Source: CAD feature listing. Evaluate the final solid. Frame: model axes, mm. A direction names the side the tool comes from. Give positions to 0.01 mm unless a question says otherwise; leave off trailing zeros. Order: outer loops, then holes, each group sorted by start corner. A loop starts at its lowest first (then second) coordinate and runs counter-clockwise, first axis right, second up.
```python
from build123d import *

# Parameters (mm, degrees)
BASE_FLANGE1_DEPTH      = 60
SKETCH6_R               = 15
CUT_EXTRUDE1_DEPTH      = 3.4
CUT_EXTRUDE2_START      = -65
CUT_EXTRUDE2_OUTLINE_W  = 10
CUT_EXTRUDE2_OUTLINE_H  = 10.4
CUT_EXTRUDE2_DEPTH      = 50
SKETCH10_W              = 3
SKETCH10_H              = 3.4
BOSS_EXTRUDE1_DEPTH     = 30
MIRROR2_COPY_1_SKETCH_W = 3
MIRROR2_COPY_1_SKETCH_H = 3.4
MIRROR2_COPY_1_DEPTH    = 30
SKETCH13_R              = 1.5
CUT_EXTRUDE3_DEPTH      = 141.516902898
CUT_EXTRUDE6_REACH      = 142.517
SKETCH14_R              = 2.5
CUT_EXTRUDE7_START      = -3.4
CUT_EXTRUDE7_DEPTH      = 10.4


# Read off the part's stored shape, not the designer's step: Cut-Extrude2
# Sheet-metal steps are written as plain solids
with BuildPart() as part:
    # Sketch1 → Base-Flange1 (new body)
    with BuildSketch(Plane.XY):
        with BuildLine():
            Line((100, 0), (4.4, 0))
            ThreePointArc((4.4, 0), (1.288730163, -1.288730163), (0, -4.4))
            Line((0, -4.4), (0, -71.6))
            ThreePointArc((0, -71.6), (1.288730163, -74.711269837), (4.4, -76))
            Line((4.4, -76), (45.6, -76))
            ThreePointArc((45.6, -76), (48.711269837, -74.711269837), (50, -71.6))
            Line((50, -71.6), (50, -70))
            ThreePointArc((50, -70), (50.292893219, -69.292893219), (51, -69))
            Line((51, -69), (100, -69))
            Line((100, -69), (100, -65.6))
            Line((100, -65.6), (51, -65.6))
            ThreePointArc((51, -65.6), (47.888730163, -66.888730163), (46.6, -70))
            Line((46.6, -70), (46.6, -71.6))
            ThreePointArc((46.6, -71.6), (46.307106781, -72.307106781), (45.6, -72.6))
            Line((45.6, -72.6), (4.4, -72.6))
            ThreePointArc((4.4, -72.6), (3.692893219, -72.307106781), (3.4, -71.6))
            Line((3.4, -71.6), (3.4, -4.4))
            ThreePointArc((3.4, -4.4), (3.692893219, -3.692893219), (4.4, -3.4))
            Line((4.4, -3.4), (100, -3.4))
            Line((100, -3.4), (100, 0))
        make_face()
    extrude(amount=BASE_FLANGE1_DEPTH)

    # Sketch6 → Cut-Extrude1 (cut)
    with BuildSketch(Plane.ZY):
        with Locations(Location((30, -50, 0), (0, 0, 270))):
            Circle(SKETCH6_R)
        with BuildLine():
            Line((57.224873734, -63.689339828), (55.810660172, -62.275126266))
            ThreePointArc((55.810660172, -62.275126266), (52.275126266, -62.275126266), (52.275126266, -65.810660172))
            Line((52.275126266, -65.810660172), (53.689339828, -67.224873734))
            ThreePointArc((53.689339828, -67.224873734), (57.224873734, -67.224873734), (57.224873734, -63.689339828))
        make_face()
        with BuildLine():
            Line((2.775126266, -16.310660172), (4.189339828, -17.724873734))
            ThreePointArc((4.189339828, -17.724873734), (7.724873734, -17.724873734), (7.724873734, -14.189339828))
            Line((7.724873734, -14.189339828), (6.310660172, -12.775126266))
            ThreePointArc((6.310660172, -12.775126266), (2.775126266, -12.775126266), (2.775126266, -16.310660172))
        make_face()
        with BuildLine():
            Line((53.689339828, -12.775126266), (52.275126266, -14.189339828))
            ThreePointArc((52.275126266, -14.189339828), (52.275126266, -17.724873734), (55.810660172, -17.724873734))
            Line((55.810660172, -17.724873734), (57.224873734, -16.310660172))
            ThreePointArc((57.224873734, -16.310660172), (57.224873734, -12.775126266), (53.689339828, -12.775126266))
        make_face()
        with BuildLine():
            Line((6.310660172, -67.224873734), (7.724873734, -65.810660172))
            ThreePointArc((7.724873734, -65.810660172), (7.724873734, -62.275126266), (4.189339828, -62.275126266))
            Line((4.189339828, -62.275126266), (2.775126266, -63.689339828))
            ThreePointArc((2.775126266, -63.689339828), (2.775126266, -67.224873734), (6.310660172, -67.224873734))
        make_face()
    extrude(amount=-CUT_EXTRUDE1_DEPTH, mode=Mode.SUBTRACT)

    # Cut-Extrude2 outline → Cut-Extrude2 (cut)
    with BuildSketch(Plane.ZY.offset(CUT_EXTRUDE2_START)):
        with Locations((55, -70.8)):
            Rectangle(CUT_EXTRUDE2_OUTLINE_W, CUT_EXTRUDE2_OUTLINE_H)
        with Locations((5, -70.8)):
            Rectangle(CUT_EXTRUDE2_OUTLINE_W, CUT_EXTRUDE2_OUTLINE_H)
    extrude(amount=CUT_EXTRUDE2_DEPTH, mode=Mode.SUBTRACT)

    # Sketch10 → Boss-Extrude1 (add)
    with BuildSketch(Plane(origin=(100, 0, 0), x_dir=(0, 0, -1), z_dir=(1, 0, 0))):
        with Locations((1.5, -1.7)):
            Rectangle(SKETCH10_W, SKETCH10_H)
    boss_extrude1 = extrude(amount=-BOSS_EXTRUDE1_DEPTH)

    # Mirror1: Boss-Extrude1 across plane
    add(boss_extrude1.mirror(Plane(origin=(0, 0, 30), x_dir=(1, 0, 0), z_dir=(0, 0, -1))))

    # Mirror2: Boss-Extrude1 across plane
    add(boss_extrude1.mirror(Plane(origin=(0, -34.5, 0), x_dir=(0, 0, 1), z_dir=(0, -1, 0))))

    # Mirror2 copy 1 sketch → Mirror2 copy 1 (add)
    with BuildSketch(Plane(origin=(100, -69, 60), x_dir=(0, 0, 1), z_dir=(1, 0, 0))):
        with Locations((1.5, -1.7)):
            Rectangle(MIRROR2_COPY_1_SKETCH_W, MIRROR2_COPY_1_SKETCH_H)
    extrude(amount=-MIRROR2_COPY_1_DEPTH)

    # Sketch13 → Cut-Extrude3 (cut, through all)
    with BuildSketch(Plane(origin=(0, 0, 0), x_dir=(1, 0, 0), z_dir=(0, 1, 0))):
        with Locations(Location((76.306667563, -8.329371406, 0), (0, 0, 270))):
            Circle(SKETCH13_R)
        with Locations(Location((93.693332437, -8.329371406, 0), (0, 0, 270))):
            Circle(SKETCH13_R)
    cut_extrude3 = extrude(amount=-CUT_EXTRUDE3_DEPTH, mode=Mode.SUBTRACT)

    # Mirror3: Cut-Extrude3 across plane
    add(cut_extrude3.mirror(Plane(origin=(0, 0, 30), x_dir=(1, 0, 0), z_dir=(0, 0, -1))), mode=Mode.SUBTRACT)

    # Sketch14 → Cut-Extrude6 (cut, up to next)
    with BuildSketch(Plane(origin=(0, 0, 0), x_dir=(1, 0, 0), z_dir=(0, 1, 0)), mode=Mode.PRIVATE) as cut_extrude6_sk1:
        with Locations(Location((20, -15, 0), (0, 0, 270))):
            Circle(SKETCH14_R)
    cut_extrude6_tool1 = extrude(cut_extrude6_sk1.sketch, amount=-CUT_EXTRUDE6_REACH, mode=Mode.PRIVATE) & part.part
    # Sketch14 → Cut-Extrude6 (cut, up to next)
    with BuildSketch(Plane(origin=(0, 0, 0), x_dir=(1, 0, 0), z_dir=(0, 1, 0)), mode=Mode.PRIVATE) as cut_extrude6_sk2:
        with Locations(Location((48, -15, 0), (0, 0, 270))):
            Circle(SKETCH14_R)
    cut_extrude6_tool2 = extrude(cut_extrude6_sk2.sketch, amount=-CUT_EXTRUDE6_REACH, mode=Mode.PRIVATE) & part.part
    # Sketch14 → Cut-Extrude6 (cut, up to next)
    with BuildSketch(Plane(origin=(0, 0, 0), x_dir=(1, 0, 0), z_dir=(0, 1, 0)), mode=Mode.PRIVATE) as cut_extrude6_sk3:
        with Locations(Location((48, -45, 0), (0, 0, 270))):
            Circle(SKETCH14_R)
    cut_extrude6_tool3 = extrude(cut_extrude6_sk3.sketch, amount=-CUT_EXTRUDE6_REACH, mode=Mode.PRIVATE) & part.part
    # Sketch14 → Cut-Extrude6 (cut, up to next)
    with BuildSketch(Plane(origin=(0, 0, 0), x_dir=(1, 0, 0), z_dir=(0, 1, 0)), mode=Mode.PRIVATE) as cut_extrude6_sk4:
        with Locations(Location((20, -45, 0), (0, 0, 270))):
            Circle(SKETCH14_R)
    cut_extrude6_tool4 = extrude(cut_extrude6_sk4.sketch, amount=-CUT_EXTRUDE6_REACH, mode=Mode.PRIVATE) & part.part
    # Sketch14 → Cut-Extrude6 (cut, up to next)
    with BuildSketch(Plane(origin=(0, 0, 0), x_dir=(1, 0, 0), z_dir=(0, 1, 0)), mode=Mode.PRIVATE) as cut_extrude6_sk5:
        with Locations(Location((34, -30, 0), (0, 0, 270))):
            Circle(SKETCH14_R)
    cut_extrude6_tool5 = extrude(cut_extrude6_sk5.sketch, amount=-CUT_EXTRUDE6_REACH, mode=Mode.PRIVATE) & part.part
    # Sketch14 → Cut-Extrude6 (cut, up to next)
    with BuildSketch(Plane(origin=(0, 0, 0), x_dir=(1, 0, 0), z_dir=(0, 1, 0)), mode=Mode.PRIVATE) as cut_extrude6_sk6:
        with Locations(Location((34, -7, 0), (0, 0, 270))):
            Circle(SKETCH14_R)
    cut_extrude6_tool6 = extrude(cut_extrude6_sk6.sketch, amount=-CUT_EXTRUDE6_REACH, mode=Mode.PRIVATE) & part.part
    # Sketch14 → Cut-Extrude6 (cut, up to next)
    with BuildSketch(Plane(origin=(0, 0, 0), x_dir=(1, 0, 0), z_dir=(0, 1, 0)), mode=Mode.PRIVATE) as cut_extrude6_sk7:
        with Locations(Location((34, -53, 0), (0, 0, 270))):
            Circle(SKETCH14_R)
    cut_extrude6_tool7 = extrude(cut_extrude6_sk7.sketch, amount=-CUT_EXTRUDE6_REACH, mode=Mode.PRIVATE) & part.part
    add(cut_extrude6_tool1.solids().sort_by_distance((20, 0, 15))[0], mode=Mode.SUBTRACT)
    add(cut_extrude6_tool2.solids().sort_by_distance((48, 0, 15))[0], mode=Mode.SUBTRACT)
    add(cut_extrude6_tool3.solids().sort_by_distance((48, 0, 45))[0], mode=Mode.SUBTRACT)
    add(cut_extrude6_tool4.solids().sort_by_distance((20, 0, 45))[0], mode=Mode.SUBTRACT)
    add(cut_extrude6_tool5.solids().sort_by_distance((34, 0, 30))[0], mode=Mode.SUBTRACT)
    add(cut_extrude6_tool6.solids().sort_by_distance((34, 0, 7))[0], mode=Mode.SUBTRACT)
    add(cut_extrude6_tool7.solids().sort_by_distance((34, 0, 53))[0], mode=Mode.SUBTRACT)

    # Sketch15 → Cut-Extrude7 (cut)
    with BuildSketch(Plane.XZ.offset(69).offset(CUT_EXTRUDE7_START)):
        Polygon((65, 50), (70, 60), (65, 60), align=None)
        Polygon((15, 50), (15, 60), (10, 60), align=None)
    cut_extrude7 = extrude(amount=CUT_EXTRUDE7_DEPTH, mode=Mode.SUBTRACT)

    # Mirror4: Cut-Extrude7 across plane
    add(cut_extrude7.mirror(Plane(origin=(0, 0, 30), x_dir=(1, 0, 0), z_dir=(0, 0, -1))), mode=Mode.SUBTRACT)


solid = part.part
```
1) Section query D-D, the plane x = 48. Return the cut outline in (y, z), and give its area (3 significant figures).
Report:
outline: (-75.29, 10) - (-66.78, 10) - (-66.78, 50) - (-75.29, 50) - close; (-3.4, 0) - (0, 0) - (0, 12.5) - (-3.4, 12.5) - close; (-3.4, 17.5) - (0, 17.5) - (0, 42.5) - (-3.4, 42.5) - close; (-3.4, 47.5) - (0, 47.5) - (0, 60) - (-3.4, 60) - close
area: 510 mm2
2) Section query A-A, the plane x = 28. Return the cut outline in (y, z), and give its area (3 significant figures).
Report:
outline: (-76, 10) - (-72.6, 10) - (-72.6, 50) - (-76, 50) - close; (-3.4, 0) - (0, 0) - (0, 60) - (-3.4, 60) - close
area: 340 mm2
3) Draft query along Z for faces 6 (the cylindrical face through (48.677, -74.745, 29.72)), 7 (the cylindrical face through (35.69, -1.68, 28.16)), 8 (the flat face through (85, -2, 63)), 9 (the cylindrical face through (93.119, -67.276, 50.285)). Return one class per face: +Z half, -Z half, draft (parallel to the pull), parting line (faces both ways), or undercut.
Report:
face 6: draft
face 7: undercut
face 8: +Z half
face 9: undercut
4) Section query C-C, the plane z = 30. Return the cut outline in (x, y), and give its area (3 significant figures).
Report:
outline: (0, -71.6) arc R4.4 ccw to (4.4, -76) - (45.6, -76) arc R4.4 ccw to (50, -71.6) - (50, -70) arc R1 cw to (51, -69) - (100, -69) - (100, -65.6) - (51, -65.6) arc R4.4 ccw to (46.6, -70) - (46.6, -71.6) arc R1 cw to (45.6, -72.6) - (4.4, -72.6) arc R1 cw to (3.4, -71.6) - (3.4, -65) - (0, -65) - close; (0, -35) - (3.4, -35) - (3.4, -4.4) arc R1 cw to (4.4, -3.4) - (31.5, -3.4) - (31.5, 0) - (4.4, 0) arc R4.4 ccw to (0, -4.4) - close; (36.5, -3.4) - (100, -3.4) - (100, 0) - (36.5, 0) - close
area: 804 mm2
5) Pin query (flat end, axial travel): pin 1 (3 mm diameter, centred on x = 47, y = -68.5, fed in from -Z); pin 2 (4 mm diameter, centred on x = 68, z = 35.5, fed in from -Y); pin 3 (8.5 mm diameter, centred on x = 32.5, y = -69, fed in from +Z). Return the tip coordinate at first contact, or that it passes through.
Report:
pin 1: stops at z = 10
pin 2: stops at y = -69
pin 3: stops at z = 50
6) Material intervals for L1, parallel to Y at x = 90, z = 40; L2, parallel to X at y = -0.85, z = 45; L3, parallel to X at y = -1, z = 7, sorted ascending.
Report:
L1: y = -69 to -65.6, -3.4 to 0
L2: x = 1.8 to 17.5, 22.5 to 45.5, 50.5 to 100
L3: x = 1.61 to 31.5, 36.5 to 75.61, 77 to 93, 94.39 to 100
7) Reachability of faces 1 (the flat face through (12.465, -74.276, 4.93)), 2 (the flat face through (70, -67, -1)), 3 (the cylindrical face through (48.1, -1.7, 12.5)), 4 (the cylindrical face through (1.68, -67.26, 57.19)), 5 (the cylindrical face through (92.36, -67.28, 9.02)) from +Z, -Z, +X, -X, +Y, -Y: full face, straight path, thin tool, end or side. Return the list, or none.
Report:
face 1: -Z, +X, -Y
face 2: -Z, -X, +Y, -Y
face 3: +Y
face 4: -X
face 5: +Y, -Y
8) Section query B-B, the plane y = -50. Return the cut outline in (x, z).
Report:
outline: (0, 0) - (3.4, 0) - (3.4, 15) - (0, 15) - close; (0, 45) - (3.4, 45) - (3.4, 60) - (0, 60) - close
